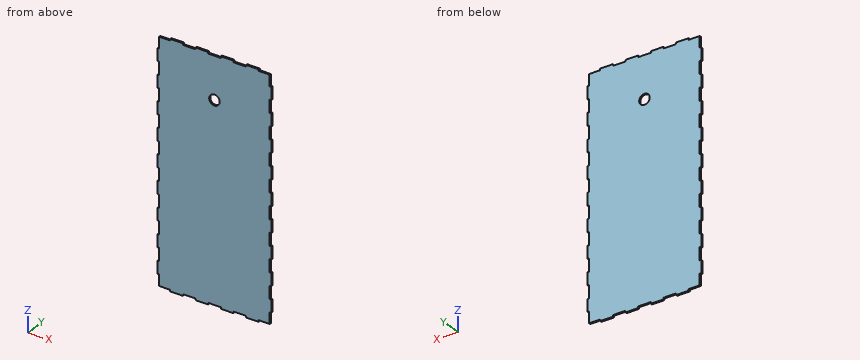
from build123d import *

# Parameters (mm, degrees)
SKETCH1_W           = 210
SKETCH1_H           = 450
SKETCH1_R           = 10
BOSS_EXTRUDE1_DEPTH = 3
SKETCH3_W           = 3
SKETCH3_H           = 24
BOSS_EXTRUDE3_DEPTH = 3
SKETCH2_W           = 24
SKETCH2_H           = 3
BOSS_EXTRUDE4_DEPTH = 3


with BuildPart() as part:
    # Sketch1 → Boss-Extrude1 (new body)
    with BuildSketch(Plane(origin=(0, 0, 0), x_dir=(1, 0, 0), z_dir=(0, 1, 0))):
        Rectangle(SKETCH1_W, SKETCH1_H)
        with Locations((0, -145)):
            Circle(SKETCH1_R, mode=Mode.SUBTRACT)
    extrude(amount=BOSS_EXTRUDE1_DEPTH)

    # Sketch3 → Boss-Extrude3 (add)
    with BuildSketch(Plane(origin=(0, 3, 0), x_dir=(1, 0, 0), z_dir=(0, 1, 0))):
        with Locations((-106.5, 192)):
            Rectangle(SKETCH3_W, SKETCH3_H)
        with Locations((106.5, 192)):
            Rectangle(SKETCH3_W, SKETCH3_H)
        with Locations((106.5, 144)):
            Rectangle(SKETCH3_W, SKETCH3_H)
        with Locations((106.5, 96)):
            Rectangle(SKETCH3_W, SKETCH3_H)
        with Locations((106.5, 48)):
            Rectangle(SKETCH3_W, SKETCH3_H)
        with Locations((106.5, 0)):
            Rectangle(SKETCH3_W, SKETCH3_H)
        with Locations((106.5, -48)):
            Rectangle(SKETCH3_W, SKETCH3_H)
        with Locations((106.5, -96)):
            Rectangle(SKETCH3_W, SKETCH3_H)
        with Locations((106.5, -144)):
            Rectangle(SKETCH3_W, SKETCH3_H)
        with Locations((106.5, -192)):
            Rectangle(SKETCH3_W, SKETCH3_H)
        with Locations((-106.5, 144)):
            Rectangle(SKETCH3_W, SKETCH3_H)
        with Locations((-106.5, 96)):
            Rectangle(SKETCH3_W, SKETCH3_H)
        with Locations((-106.5, 48)):
            Rectangle(SKETCH3_W, SKETCH3_H)
        with Locations((-106.5, 0)):
            Rectangle(SKETCH3_W, SKETCH3_H)
        with Locations((-106.5, -48)):
            Rectangle(SKETCH3_W, SKETCH3_H)
        with Locations((-106.5, -96)):
            Rectangle(SKETCH3_W, SKETCH3_H)
        with Locations((-106.5, -144)):
            Rectangle(SKETCH3_W, SKETCH3_H)
        with Locations((-106.5, -192)):
            Rectangle(SKETCH3_W, SKETCH3_H)
    extrude(amount=-BOSS_EXTRUDE3_DEPTH)

    # Sketch2 → Boss-Extrude4 (add)
    with BuildSketch(Plane(origin=(0, 3, 0), x_dir=(1, 0, 0), z_dir=(0, 1, 0))):
        with Locations((-72, 226.5)):
            Rectangle(SKETCH2_W, SKETCH2_H)
        with Locations((-24, 226.5)):
            Rectangle(SKETCH2_W, SKETCH2_H)
        with Locations((24, 226.5)):
            Rectangle(SKETCH2_W, SKETCH2_H)
        with Locations((72, 226.5)):
            Rectangle(SKETCH2_W, SKETCH2_H)
        with Locations((-71.999992639, -226.5)):
            Rectangle(SKETCH2_W, SKETCH2_H)
        with Locations((-23.999992639, -226.5)):
            Rectangle(SKETCH2_W, SKETCH2_H)
        with Locations((24.000007361, -226.5)):
            Rectangle(SKETCH2_W, SKETCH2_H)
        with Locations((72.000007361, -226.5)):
            Rectangle(SKETCH2_W, SKETCH2_H)
    extrude(amount=-BOSS_EXTRUDE4_DEPTH)


solid = part.part
Can you work these out from the model? Positions are in its coordinate system, mm. Round coordinates to 2 decimals unless told otherwise and drop trailing zeros. Order: outer loops, then holes, each group sorted by start corner. A loop starts at its lowest first (then second) coordinate and runs counter-clockwise, first axis right, second up. Notation, with made-up numbers: (9, -12.5) -> (45, -12.5) arc R20 ccw to (45, -5.5) -> close; hole circle Ø10 at (22, -8). An arc over 180 degrees is marked (long way). Write each question's results on one line, items separated by ' | '. Start each with the question number.
Item 1: If we section it at C-C, the plane z = -69: Write out the boundary of the cut face in (x, y), then the cut area to 3 significant figures.
Item 2: If we section it at B-B, the plane x = 0: Write out the boundary of the cut face in (y, z), then the cut area to 3 significant figures.
Item 3: Please list where these lines run through material, in increasing order: L1, parallel to X at y = 1.7, z = 145; L2, parallel to Z at x = 0, y = 1.75; L3, parallel to X at y = 2.1, z = -165.
Item 4: If we section it at A-A, the plane z = 145: Write out the boundary of the cut face in (x, y).
Item 5: Will these pins go through, and if not, where does the flat tip stop? pin 1 (8 mm diameter, centred on x = 4, z = -88, fed in from -Y); pin 2 (1.5 mm diameter, centred on x = 107, y = 1, fed in from -Z); pin 3 (0.9 mm diameter, centred on y = 1.5, z = 226, fed in from +X); pin 4 (0.9 mm diameter, centred on x = 91.5, y = 2, fed in from -Z).
Results:
1) outline: (-105, 0) -> (105, 0) -> (105, 3) -> (-105, 3) -> close | area: 630 mm2
2) outline: (0, -225) -> (3, -225) -> (3, 135) -> (0, 135) -> close; (0, 155) -> (3, 155) -> (3, 225) -> (0, 225) -> close | area: 1,290 mm2
3) L1: x = -108 to -10, 10 to 108 | L2: z = -225 to 135, 155 to 225 | L3: x = -105 to 105
4) outline: (-108, 0) -> (-10, 0) -> (-10, 3) -> (-108, 3) -> close; (10, 0) -> (108, 0) -> (108, 3) -> (10, 3) -> close
5) pin 1: stops at y = 0 | pin 2: stops at z = -204 | pin 3: stops at x = 84 | pin 4: stops at z = -225
